```python
from build123d import *

# Parameters (mm, degrees)
F0_R     = 74.6125
F1_DEPTH = 9.525
F2_R     = 15.875
F3_DEPTH = 9.526
F5_D     = 5.4
F6_R     = 2.7
F7_DEPTH = 9.526
F9_D     = 7.2


with BuildPart() as f1:
    # F0 (on Top) → F1 (new body)
    with BuildSketch(Plane.XY):
        Circle(F0_R)
    extrude(amount=F1_DEPTH)

    # F2 (on face) → F3 (cut, through all)
    with BuildSketch(Plane.XY.offset(9.525)):
        Circle(F2_R)
    extrude(amount=-F3_DEPTH, mode=Mode.SUBTRACT)

    # F5 (through all)
    with Locations(Plane.XY.offset(9.525)):
        with Locations((-13.3652133, 32.2664949823), (-32.2664903636, 13.3652244507), (-32.2664949823, -13.3652133), (-13.3652244507, -32.2664903636), (13.3652133, -32.2664949823), (32.2664903636, -13.3652244507), (32.2664949823, 13.3652133), (13.3652244507, 32.2664903636)):
            Hole(F5_D / 2)

    # F6 (on face) → F7 (cut, through all)
    with BuildSketch(Plane.XY.offset(9.525)):
        with BuildLine():
            Line((92.0014753938, 88.4870588779), (0, 88.4870588779))
            Line((0, 88.4870588779), (0, 74.6125))
            ThreePointArc((0, 74.6125), (52.7590047113, 52.7590047113), (74.6125, 0))
            ThreePointArc((74.6125, 0), (52.7590047113, -52.7590047113), (0, -74.6125))
            Line((0, -74.6125), (0, -93.3939293027))
            Line((0, -93.3939293027), (92.0014753938, -93.3939293027))
            Line((92.0014753938, -93.3939293027), (92.0014753938, 88.4870588779))
        make_face()
        with BuildLine():
            ThreePointArc((74.6125, 0), (52.7590047113, 52.7590047113), (0, 74.6125))
            Line((0, 74.6125), (0, 15.875))
            ThreePointArc((0, 15.875), (11.2253201513, 11.2253201513), (15.875, 0))
            ThreePointArc((15.875, 0), (11.2253201513, -11.2253201513), (0, -15.875))
            Line((0, -15.875), (0, -74.6125))
            ThreePointArc((0, -74.6125), (52.7590047113, -52.7590047113), (74.6125, 0))
        make_face()
        with Locations((13.3652133, -32.2664949823)):
            Circle(F6_R, mode=Mode.SUBTRACT)
        with Locations((32.2664903636, -13.3652244507)):
            Circle(F6_R, mode=Mode.SUBTRACT)
        with Locations((32.2664949823, 13.3652133)):
            Circle(F6_R, mode=Mode.SUBTRACT)
        with Locations((13.3652244507, 32.2664903636)):
            Circle(F6_R, mode=Mode.SUBTRACT)
    extrude(amount=-F7_DEPTH, mode=Mode.SUBTRACT)

    # F9 (through all)
    with Locations(Plane.XY.offset(9.525)):
        with Locations((-24.300392725, 58.6663524809), (-58.6663481481, 24.3004031854), (-58.6663524809, -24.300392725), (-24.3004031854, -58.6663481481)):
            Hole(F9_D / 2)


solid = f1.part
```
Design review of the part built by this model. Coordinates are the model's own, in mm. Give positions to 0.01 mm unless a question says otherwise; leave off trailing zeros. Order: outer loops, then holes, each group sorted by start corner. A loop starts at its lowest first (then second) coordinate and runs counter-clockwise, first axis right, second up. Notation, with made-up numbers: M 45,78.25 L 53,78.25 A19 ccw 53,102.25 Z; hole C 43,84 d3. An arc over 180 degrees is marked long. One line per question, with ' | ' between items. Start each with the question number.
Q1. We need section A-A (z = 7). State how many separate pieces and enclosed holes the cut face has, plus the area to 3 significant figures.
Q2. For pin 1 Ø4 at (y, z) = (6.5, 7) entering from -X; pin 2 Ø5 at (x, z) = (-13, 8.5) entering from +Y; pin 3 Ø1.5 at (y, z) = (-9.5, 6) entering from +X; pin 4 Ø6 at (x, y) = (-24.3, -58.67) entering from +Z, all flat-tipped, find the tip position at first contact; note any pin that passes through.
Q3. We need section C-C (x = -41). Write out the cut boundary in (y, z) (3 decimals).
Q4. We need section B-B (y = 0). Write out the cut boundary in (x, z) (1 decimal).
Q5. The part is to be moulded in two halves that separate along Y. For faces 1 (the face through (-15.87, 0.35, 4.83)), 2 (the face through (-74.594, 1.641, 4.696)), 3 (the face through (0, 46, 5)), say which applies: +Y half, -Y half, draft (parallel to the pull), parting line (faces both ways), or undercut.
Q6. For L1, parallel to Y at x = -27.5, z = 3.25; L2, parallel to Y at x = -23, z = 8; L3, parallel to Y at x = -13.5, z = 5.75, list the stretches that pass through material, from the lowest coordinate up. Write a range as [from, to].
Returned:
1) separate pieces: 1 | enclosed holes: 8 | area: 8,090 mm2
2) pin 1: x = -74.48 | pin 2: y = 73.87 | pin 3: x = -12.12 | pin 4: through
3) outline: M -62.338,0 L 62.338,0 L 62.338,9.525 L -62.338,9.525 Z
4) outline: M -74.6,0 L -15.9,0 L -15.9,9.5 L -74.6,9.5 Z
5) face 1: undercut | face 2: parting line | face 3: draft
6) L1: [-69.36, -60.32], [-57.02, 57.02], [60.32, 69.36] | L2: [-70.98, -62.02], [-55.31, 55.31], [62.02, 70.98] | L3: [-73.38, -34.96], [-29.57, -8.35], [8.35, 29.57], [34.96, 73.38]
